Could you check a few things on this drawing? It's one solid part, dimensions in mm from its lowest x, y, z. A direction names the side the tool comes from. Coordinates: 2 decimals unless noted, no trailing zeros. Write each loop counter-clockwise with the first axis right and the second up, starting at its lowest first coordinate (ties: lowest second). Pieces come first, ordered by that corner, then holes.
Item 1: I want a section at B-B (x = 33.5). Please give me the cut outline in (y, z), and give its area (3 significant figures).
Item 2: If we mould it in two halves opening along Y, with no side actions, what happens to the marked faces 3, 4 and 5? For each: pulls with the +Y half, pulls with the -Y half, needs draft (parallel to the pull), parting line crosses it, or undercut.
Item 3: Please list where these lines run through material, in increasing order: line 1 (Y direction, x = 40, z = 6) (1 decimal); line 2 (X direction, y = 27, z = 10) (1 decimal); line 3 (Y direction, x = 34, z = 3).
Item 4: I'm going to push flat-ended pins straight in: P1, Ø6, axis at x = 19, y = 47, coming from the -Z side; P2, Ø6, axis at y = 23, z = 3.5, coming from the +X side (1 decimal); P3, Ø7.5, axis at y = 35, z = 10.5, coming from the +X side; P4, Ø12.5, axis at x = 36, z = 18, coming from the -Y side. Where does each tip first touch, or does it pass through?
Item 5: I want a section at D-D (y = 21). Please give me the cut outline in (x, z), and give its area (3 significant figures).
Item 6: I want a section at C-C (z = 3). Please give me the cut outline in (x, y), and give its area (3 significant figures).
Item 7: For the marked faces 1 and 2, which set-ups out of +Z, -Z, +X, -X, +Y, -Y let a thin tool reach every point of the face, with its end or its side?
Item 8: I want a section at A-A (y = 32). Please give me the cut outline in (x, z), and give its area (3 significant figures).
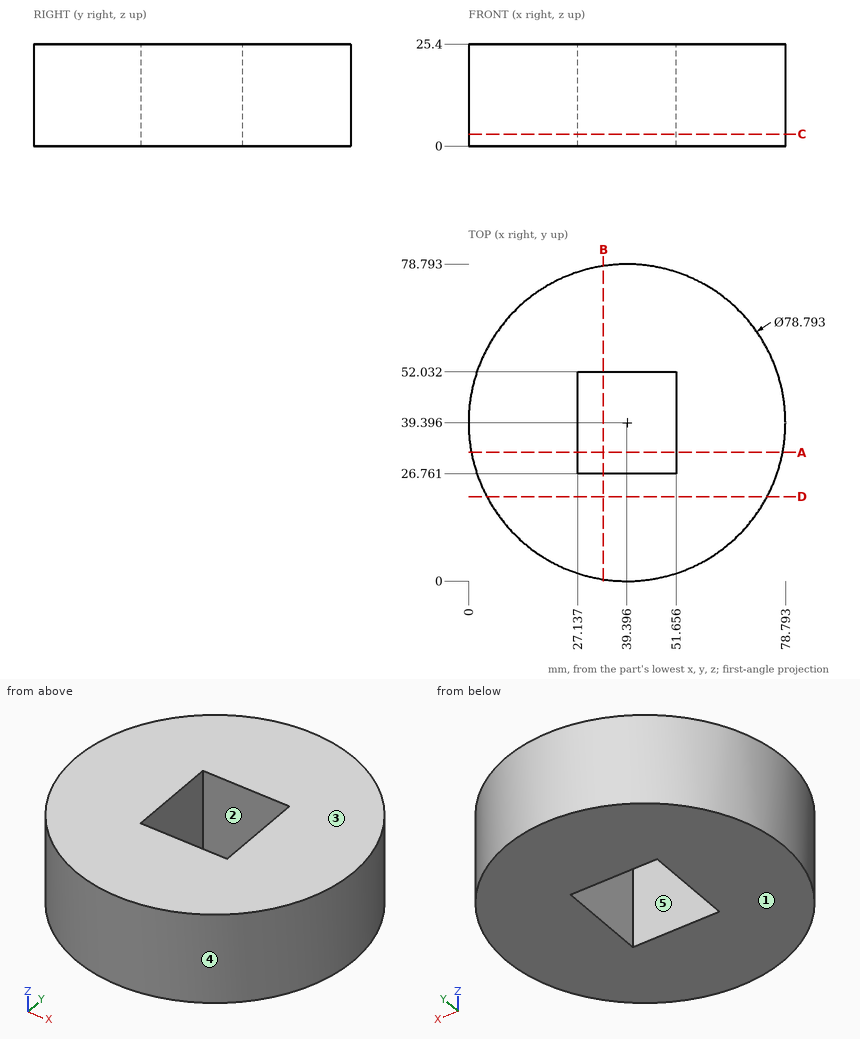
Answer:
1. outline: (0.44, 0) - (26.76, 0) - (26.76, 25.4) - (0.44, 25.4) - close; (52.03, 0) - (78.35, 0) - (78.35, 25.4) - (52.03, 25.4) - close
1. area: 1,340 mm2
2. face 3: needs draft
2. face 4: parting line crosses it
2. face 5: undercut
3. line 1: y = 0 to 26.8, 52 to 78.8
3. line 2: x = 2 to 27.1, 51.7 to 76.8
3. line 3: y = 0.37 to 26.76, 52.03 to 78.42
4. P1: stops at z = 0
4. P2: stops at x = 76.4
4. P3: stops at x = 78.79
4. P4: stops at y = 0
5. outline: (4.56, 0) - (74.23, 0) - (74.23, 25.4) - (4.56, 25.4) - close
5. area: 1,770 mm2
6. outline: circle Ø78.79 at (39.4, 39.4); hole (27.14, 26.76) - (51.66, 26.76) - (51.66, 52.03) - (27.14, 52.03) - close
6. area: 4,260 mm2
7. face 1: -Z, +X, -X, +Y, -Y
7. face 2: +Z, -Z
8. outline: (0.7, 0) - (27.14, 0) - (27.14, 25.4) - (0.7, 25.4) - close; (51.66, 0) - (78.09, 0) - (78.09, 25.4) - (51.66, 25.4) - close
8. area: 1,340 mm2
